Here's how the part is built. I have some questions about the finished solid (model axes, mm). A direction names the side the tool comes from. Coordinates: 2 decimals unless noted, no trailing zeros. Write each loop counter-clockwise with the first axis right and the second up, starting at its lowest first coordinate (ties: lowest second). Pieces come first, ordered by that corner, then holes. Notation, with made-up numbers: M 45.25,45 L 64.25,45 A31 ccw 64.25,73 Z; hole C -8,-35 d8. An arc over 180 degrees is marked long. Use one line per item in the form item = value. Start each with the question number.
1. I want a section at B-B, the plane y = 6.35. List the corners of the cut face in (x, z) for me (3 decimals).
2. I want a section at C-C, the plane z = 0. List the corners of the cut face in (x, y) for me (3 decimals), plus the area to 3 significant figures.
3. Thinking about a two-plate mould opening in Z: for faces 1 (the face through (-29.25, 6.26, 3.75)), 2 (the face through (-22, 12.7, 0)), 3 (the face through (-31.65, 4.468, 0.137)), which applies, released by +Z, released by -Z, zero draft, split by the parting line, or undercut?
4. I want a section at A-A, the plane z = -2.25. List the corners of the cut face in (x, y) for me (3 decimals), plus the area to 3 significant figures.
5. On a 3-axis mill with a long thin cutter (end or side, diameter ignored), from which of +Z, -Z, +X, -X, +Y, -Y can I reach the whole of each face in a straight line? I mean faces 4 (the face through (-9.246, 6, 0)), 5 (the face through (-12.61, 5.57, 0.1)). Say none if no direction works.
6. I want a section at D-D, the plane z = 1.25. List the corners of the cut face in (x, y) for me (3 decimals), plus the area to 3 significant figures.
7. Please list where these lines run through material, in increasing order: line 1 along X through (y, z) = (6.25, 0) (3 decimals); line 2 along X through (y, z) = (2.75, 0) (3 decimals); line 3 along Y through (x, z) = (-12.25, 0). Write a range as [from, to].
8. I'm going to push flat-ended pins straight in: pin 1 Ø2 at (x, y) = (-15, 4) entering from -Z; pin 2 Ø5 at (x, y) = (-29.5, 9.5) entering from +Z; pin 3 Ø1.5 at (y, z) = (5.5, 2) entering from -X. Where does each tip first touch, or does it pass through?
Autodesk Inventor part; units mm, degrees
ref_plane "Work Plane1" through (-32.385, 0, 0) normal (1, 0, 0) x (0, 1, 0)
ref_plane "YZ Plane" through (0, 0, 0) normal (1, 0, 0) x (0, 1, 0)
ref_plane "XZ Plane" through (0, 0, 0) normal (0, 1, 0) x (-1, 0, 0)
sketch "Sketch1" plane through (0, 0, 0) normal (0, 1, 0) x (-1, 0, 0)
  line L0 (0, 0) -> (28.575, 0)
  line L1 (28.575, 0) -> (0, 0)
  line L2 (0, 0) -> (-14.2875, -24.7467)
  line L3 (0, 0) -> (28.575, 0) construction
  line L4 (0, 0) -> (-14.2875, 24.7467)
  line L5 (0, 0) -> (28.575, 0) construction
  circle A0 centre (28.575, 0) radius 2.54
  circle A1 centre (-14.2875, -24.7467) radius 2.54
  circle A2 centre (-14.2875, 24.7467) radius 2.54
  circle A3 centre (0, 0) radius 3.175
  circle A4 centre (0, 0) radius 6.35
  line L6 (-1.5875, -2.7496) -> (0, 0)
  line L7 (0, 0) -> (-6.35, 0)
  circle A5 centre (-14.2875, 24.7467) radius 3.81
  circle A6 centre (28.575, 0) radius 3.81
  circle A7 centre (-14.2875, -24.7467) radius 3.81
  line L8 (30.6811, 3.175) -> (-12.1814, 27.9217)
  line L9 (28.2054, -3.792) -> (-10.8187, -26.3226)
  line L10 (-18.0975, 24.7467) -> (-18.0975, -24.7467)
  line L11 (0, 0) -> (5.0525, -8.8146)
  line L12 (0, 0) -> (5.1463, 8.7602)
  line L13 (0, 0) -> (-10.16, 0)
  arc A8 (28.2054, -3.792) -> (-10.8187, -26.3226) centre (24.4473, -42.344) ccw
  arc A9 (-10.8187, 26.3226) -> (28.2054, 3.792) centre (24.4473, 42.344) ccw
  arc A10 (-17.3867, -22.5305) -> (-17.3867, 22.5305) centre (-48.8947, 0) ccw
  point P0 (5.1074, 8.7829)
  point P1 (-10.16, 0.0317)
  point P2 (30.2716, 3.4114)
  point P3 (28.2054, 3.792)
  point P4 (-10.8187, 26.3226)
  point P5 (-17.3867, 22.5305)
  point P6 (-17.3867, -22.5305)
  dimension "d9" = 6.35
  dimension "d41" = 12.7
  dimension "d0" = 28.575
  dimension "d1" = 28.575
  dimension "d2" = 120
  dimension "d3" = 28.575
  dimension "d4" = 120
  dimension "d5" = 5.08
  dimension "d6" = 5.08
  dimension "d7" = 5.08
  dimension "d42" = 7.62
  dimension "d43" = 7.62
  dimension "d44" = 7.62
  dimension "d47" = 10.16
  dimension "d48" = 10.16
  dimension "d49" = 10.16
  dimension "d52" = 360
extrude "Extrusion4" add sketch "Sketch1" along normal blind 12.7 contours A3 L12 A4 L0 | L0 A4 L11 A3 | A3 L11 A4 L2 | L2 A4 L7 A3 | A3 L7 A4 L4 | L4 A4 L12 A3 | A4 L12 A9 A6 L0 | L0 A6 A8 L11 A4 | A4 L11 A8 A7 L2 | L2 A7 A10 L13 A4 | A4 L13 A10 A5 L4 | L4 A5 A9 L12 A4 | A6 L8 | A7 | A5 picked at (31.8987, 0.5122)
sketch "Sketch8" plane through (0, 12.7, 0) normal (0, 1, 0) x (1, 0, 0)
  circle A0 centre (0.678, -11.6167) radius 3.175
  circle A1 centre (9.1268, -7.2186) radius 3.175
  circle A2 centre (0.678, -11.6167) radius 3.175
  circle A3 centre (9.1268, -7.2186) radius 3.175
  line L0 (5.0649, -17.2561) -> (12.4117, -13.0144)
  arc A4 (17.3867, 22.5305) -> (17.3867, -22.5305) centre (48.8947, 0) ccw
  circle A5 centre (14.2875, -24.7467) radius 2.54
  line L1 (0, 0) -> (14.2875, -24.7467)
  arc A6 (10.8187, -26.3226) -> (-28.2054, -3.792) centre (-24.4473, -42.344) ccw
  arc A7 (10.8187, -26.3226) -> (17.3867, -22.5305) centre (14.2875, -24.7467) ccw
  line L2 (9.1268, -7.2186) -> (10.7143, -9.9682)
  line L3 (9.1268, -7.2186) -> (7.5393, -4.4689)
  line L4 (0.678, -11.6167) -> (-0.9095, -8.867)
  line L5 (0.678, -11.6167) -> (2.2655, -14.3663)
  line L6 (-0.9095, -8.867) -> (-4.4671, -10.921)
  line L7 (2.2655, -14.3663) -> (-2.6369, -17.1967)
  line L8 (7.5393, -4.4689) -> (12.4407, -1.6391)
  line L9 (10.7143, -9.9682) -> (17.8581, -5.8438)
  point P0 (11.3663, -9.5918)
  point P1 (11.3414, -9.4937)
  point P2 (10.4005, -4.3102)
  point P3 (10.2682, -2.8934)
  point P4 (-0.9095, -8.867)
  point P5 (-3.012, -10.0809)
  point P6 (2.1732, -14.2063)
extrude "Extrusion5" cut sketch "Sketch8" against normal through all contours A0 A6 L5 L4 | L4 L5 A6 A0 | A0 A6 L6 | A0 L5 A6 | L3 L2 A1 | L8 A4 A1 | A1 A4 L2 L3 | A1 A4 L9 | A1 A4 picked at (2.2194, -14.2744)
sketch "Sketch11" plane through (0, 12.7, 0) normal (0, 1, 0) x (1, 0, 0)
  arc A0 (10.8187, -26.3226) -> (2.3124, -14.3387) centre (-24.4473, -42.344) ccw
  arc A1 (11.3663, -9.5918) -> (17.3867, -22.5305) centre (48.8947, 0) ccw
  arc A2 (10.8187, -26.3226) -> (17.3867, -22.5305) centre (14.2875, -24.7467) ccw
  line L0 (0, 0) -> (14.2875, -24.7467)
  circle A3 centre (14.2875, -24.7467) radius 2.54
  line L1 (14.2875, -24.7467) -> (8.2579, -14.3032)
  line L2 (14.2875, -24.7467) -> (7.9375, -13.7482)
  line L3 (7.9375, -13.7482) -> (11.895, -11.4633)
  line L4 (7.9375, -13.7482) -> (3.98, -16.033)
  circle A4 centre (14.2875, 24.7467) radius 2.54
  line L5 (0, 0) -> (14.2875, 24.7467)
  line L6 (14.2875, 24.7467) -> (7.9375, 13.7482)
  line L7 (7.9375, 13.7482) -> (0, 0)
  circle A5 centre (-28.575, 0) radius 2.54
  line L8 (0, 0) -> (-28.575, 0)
  line L9 (-28.575, 0) -> (-15.875, 0)
  line L10 (-15.875, 0) -> (-15.875, 4.5698)
  arc A6 (-28.2054, 3.792) -> (10.8187, 26.3226) centre (-24.4473, 42.344) ccw
  line L11 (-15.875, 0) -> (-15.875, -4.5698)
  line L12 (7.9375, 13.7482) -> (3.98, 16.033)
  line L13 (7.9375, 13.7482) -> (11.895, 11.4633)
  arc A7 (17.3867, 22.5305) -> (10.2682, -2.8934) centre (48.8947, 0) ccw
  arc A8 (-28.2054, 3.792) -> (-30.6811, -3.175) centre (-28.575, 0) ccw
  arc A9 (-3.012, -10.0809) -> (-28.2054, -3.792) centre (-24.4473, -42.344) ccw
  arc A10 (-30.2716, -3.4114) -> (-28.2054, -3.792) centre (-28.575, 0) ccw
  line L14 (-30.6811, -3.175) -> (-30.2716, -3.4114)
  arc A11 (17.3867, 22.5305) -> (10.8187, 26.3226) centre (14.2875, 24.7467) ccw
  line L15 (-3.012, -10.0809) -> (-0.9095, -8.867)
  arc A12 (2.3124, -14.3387) -> (-0.9095, -8.867) centre (0.678, -11.6167) ccw
  arc A13 (7.5393, -4.4689) -> (10.7143, -9.9682) centre (9.1268, -7.2186) ccw
  line L16 (11.3663, -9.5918) -> (10.7143, -9.9682)
  line L17 (7.5393, -4.4689) -> (10.2682, -2.8934)
  dimension "d65" = 12.7
  dimension "d66" = 12.7
  dimension "d67" = 12.7
extrude "Extrusion6" cut sketch "Sketch11" against normal blind 12.7 contours A0 A12 L15 A9 L11 L8 L0 L4 | L0 L5 L13 A7 L17 A13 L16 A1 L3 | L8 L10 A6 L12 L5
sketch "Sketch13" plane through (0, 12.7, 0) normal (0, 1, 0) x (1, 0, 0)
  arc A0 (-28.2054, 3.792) -> (-15.875, 4.5698) centre (-24.4473, 42.344) ccw
  arc A1 (-15.875, -4.5698) -> (-28.2054, -3.792) centre (-24.4473, -42.344) ccw
  line L0 (-15.875, -4.5698) -> (-15.875, 4.5698)
  arc A2 (-30.2716, -3.4114) -> (-28.2054, -3.792) centre (-28.575, 0) ccw
  arc A3 (-28.2054, 3.792) -> (-30.6811, -3.175) centre (-28.575, 0) ccw
  arc A4 (17.3867, 22.5305) -> (11.895, 11.4633) centre (48.8947, 0) ccw
  line L1 (3.98, 16.033) -> (11.895, 11.4633)
  arc A5 (3.98, 16.033) -> (10.8187, 26.3226) centre (-24.4473, 42.344) ccw
  arc A6 (17.3867, 22.5305) -> (10.8187, 26.3226) centre (14.2875, 24.7467) ccw
  arc A7 (11.895, -11.4633) -> (17.3867, -22.5305) centre (48.8947, 0) ccw
  line L2 (11.895, -11.4633) -> (3.98, -16.033)
  arc A8 (10.8187, -26.3226) -> (3.98, -16.033) centre (-24.4473, -42.344) ccw
  arc A9 (10.8187, -26.3226) -> (17.3867, -22.5305) centre (14.2875, -24.7467) ccw
  point P0 (0, 0)
extrude "Extrusion7" cut sketch "Sketch13" against normal blind 12.7
sketch "Sketch14" plane through (-15.875, 12.7, 4.5698) normal (1, 0, 0) x (0, 0, -1)
  line L0 (0, -12.7) -> (0, 0)
  line L1 (0, -6.35) -> (9.1395, -6.35)
  line L2 (9.1395, 0) -> (9.1395, -12.7)
  line L3 (2.0298, 0) -> (7.1098, 0)
  line L4 (4.5698, 0) -> (4.5698, -12.7)
  circle A0 centre (4.5698, -6.35) radius 0.7876
extrude "Extrusion8" add sketch "Sketch14" along normal blind 6.6294
thread "Thread1"
ref_plane "Work Plane1" through (-32.385, 0, 0) normal (1, 0, 0) x (0, 1, 0)
sketch "Sketch23" plane through (-32.385, 0, 0) normal (1, 0, 0) x (0, 1, 0)
  point P0 (0, 0)
  point P1 (5.1729, 0.2292)
hole "Hole5" at (-32.385, 5.1729, 0.2292) direction (1, 0, 0) diameter 1.4211 depth 5.715
properties part number "backupstability"
Answer list:
q1.outline = M -30.681,3.175 A3.81 ccw -28.205,-3.792 A38.735 cw -15.875,-4.57 L -15.875,-0.788 L -9.246,-0.788 L -9.246,0.788 L -15.875,0.788 L -15.875,4.57 A38.735 cw -28.205,3.792 A3.81 ccw -30.272,3.411 Z; hole C -28.575,0 d5.08
q2.outline = M -32.385,0 L -31.115,0 L -31.115,4.5 L -32.385,4.5 Z; M -32.385,5.845 L -31.115,5.845 L -31.115,12.7 L -32.385,12.7 Z; M -26.035,0 L -15.875,0 L -15.875,5.562 L -9.246,5.562 L -9.246,7.138 L -15.875,7.138 L -15.875,12.7 L -26.035,12.7 Z
q2.area = 154 mm²
q3.face_1 = released by +Z
q3.face_2 = zero draft
q3.face_3 = undercut
q4.outline = M -31.65,0 L -29.754,0 L -29.754,12.7 L -31.65,12.7 Z; M -27.396,0 L -15.875,0 L -15.875,12.7 L -27.396,12.7 Z
q4.area = 170 mm²
q5.face_4 = +Z, -Z, +X, +Y, -Y
q5.face_5 = +X
q6.outline = M -32.174,0 L -30.786,0 L -30.786,12.7 L -32.174,12.7 Z; M -26.364,0 L -15.875,0 L -15.875,12.7 L -26.364,12.7 Z
q6.area = 151 mm²
q7.line_1 = [-32.385, -31.115], [-26.035, -9.246]
q7.line_2 = [-32.385, -31.115], [-26.035, -15.875]
q7.line_3 = [5.56, 7.14]
q8.pin_1 = -4.57
q8.pin_2 = 3.81
q8.pin_3 = -32.17
